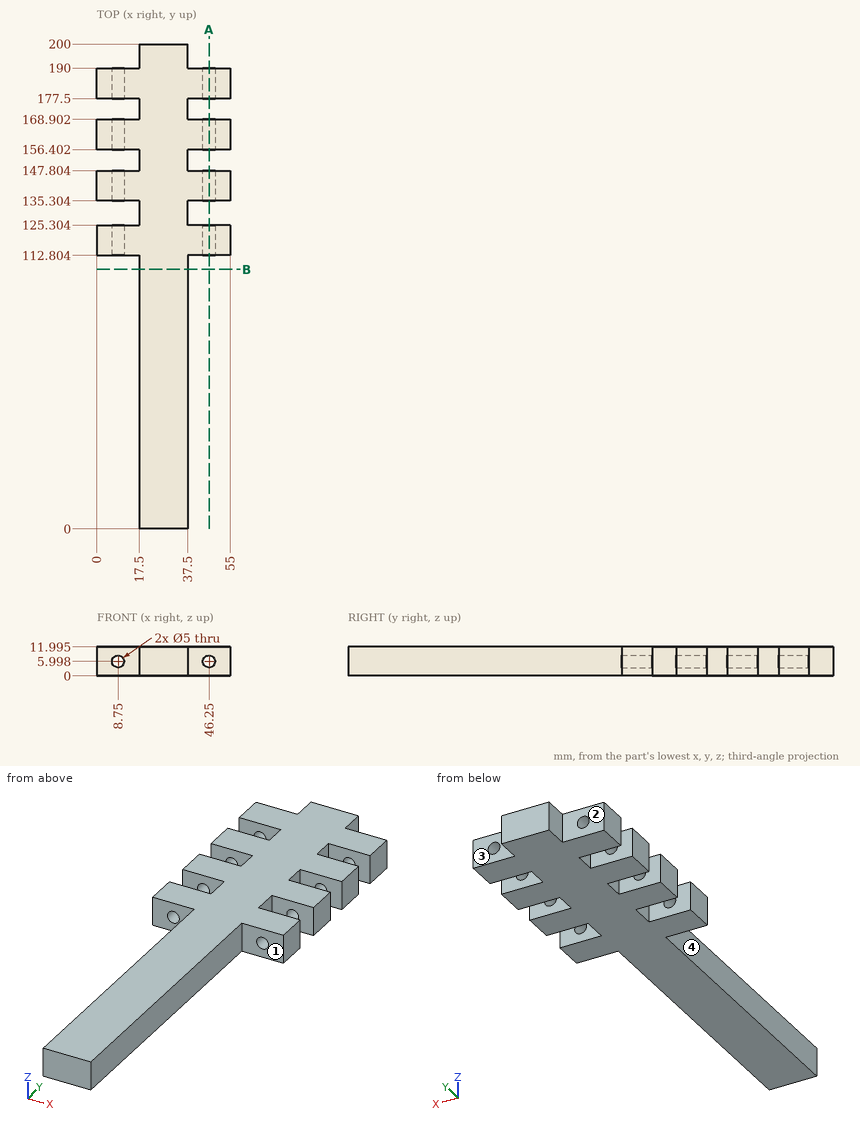
Input: dimensioned drawing with shaded views. Units: mm. Origin: part minimum x, y, z. A direction names the side the tool comes from. Give positions to 0.01 mm unless a question says otherwise; leave off trailing zeros. Write each loop counter-clockwise with the first axis right and the second up, starting at its lowest first coordinate (ties: lowest second). Pieces come first, ordered by that corner, then holes.
Q1. First-contact query: P1, Ø10, axis at x = 14.5, y = 28, coming from the -Z side; P2, Ø2.5, axis at y = 172.5, z = 8, coming from the -X side; P3, Ø4, axis at x = 49.5, z = 9.5, coming from the -Y side. Flat tips, straight axial feed; report the tip coordinate or a pass-through.
Q2. Material intervals for probe 1 along Y at (x, z) = (49, 9.5); probe 2 along Z at (x, y) = (46, 161) (1 decimal); probe 3 along X at (y, z) = (22, 0.5), sorted ascending.
Q3. Section B-B, the plane y = 107. Output: boundary loops of the cut face in (x, z) (1 decimal), plus the area to 3 significant figures.
Q4. Set-up query: the marked faces 1, 2, 3 and 4. Return all of +Z, -Z, +X, -X, +Y, -Y with unobstructed straight access to the full face (end or side cutting, diameter ignored); none if empty.
Q5. Section A-A, the plane x = 46.25. State how many separate pieces and enclosed holes the cut face has.
Filled in:
1. P1: stops at z = 0
1. P2: stops at x = 17.5
1. P3: stops at y = 112.8
2. probe 1: y = 112.8 to 125.3, 135.3 to 147.8, 156.4 to 168.9, 177.5 to 190
2. probe 2: z = 0 to 3.5, 8.5 to 12
2. probe 3: x = 17.5 to 37.5
3. outline: (17.5, 0) - (37.5, 0) - (37.5, 12) - (17.5, 12) - close
3. area: 240 mm2
4. face 1: +Z, -Z, +X, -Y
4. face 2: +Z, -Z, -X, +Y
4. face 3: +Z, -Z, +X, +Y
4. face 4: +Z, -Z, -X, -Y
5. separate pieces: 8
5. enclosed holes: 0
